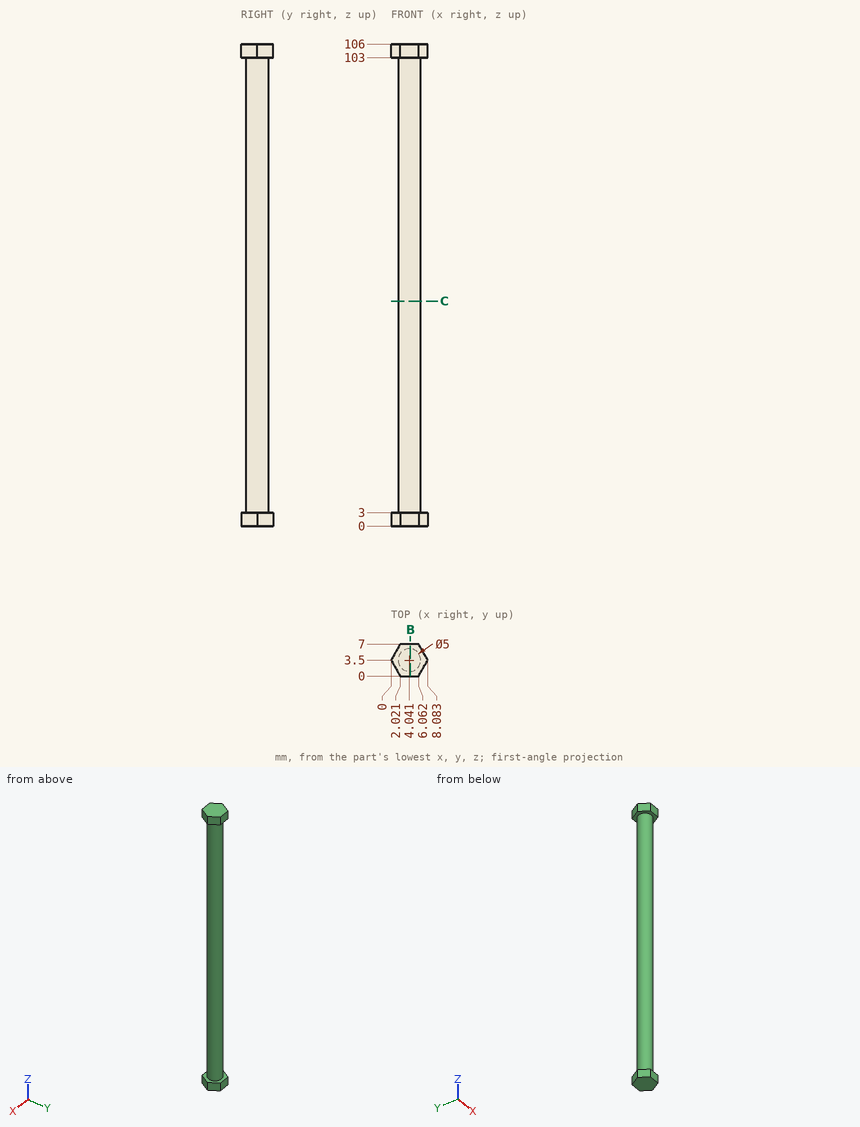
Design review of the part shown in the three views and the two pictorial views. Dimensions are in mm from the part's minimum x, y and z. Round coordinates to 2 decimals unless told otherwise and drop trailing zeros. Write each loop counter-clockwise with the first axis right and the second up, starting at its lowest first coordinate (ties: lowest second). Pieces come first, ordered by that corner, then holes.
Item 1: For pin 1 Ø2 at (y, z) = (3, 42) entering from -X; pin 2 Ø1 at (x, z) = (1.5, 83) entering from -Y (1 decimal), all flat-tipped, find the tip position at first contact; note any pin that passes through.
Item 2: Consider section B-B on x = 4.25. Give the boundary of the cut face in (y, z), and give its area (3 significant figures).
Item 3: Wall thickness on L1, parallel to Z at x = 3, y = 6; L2, parallel to Y at x = 3.75, z = 98.5; L3, parallel to X at y = 5, z = 23: over which ranges is each line inside the solid? List them lowest first.
Item 4: Consider section C-C on z = 49.5. Give the boundary of the cut face in (x, y).
Check values:
1. pin 1: stops at x = 1.54
1. pin 2: stops at y = 2.1
2. outline: (0, 0) - (7, 0) - (7, 3) - (5.99, 3) - (5.99, 103) - (7, 103) - (7, 106) - (0, 106) - (0, 103) - (1.01, 103) - (1.01, 3) - (0, 3) - close
2. area: 540 mm2
3. L1: z = 0 to 3, 103 to 106
3. L2: y = 1.02 to 5.98
3. L3: x = 2.04 to 6.04
4. outline: circle Ø5 at (4.04, 3.5)
